Geometry: final body of the model. Coordinates: model frame, mm. Face numbers are marked on the shaded views. A direction names the side the tool comes from. Give positions to 0.01 mm unless a question says otherwise; leave off trailing zeros. Loops run counter-clockwise (first coordinate to the right, second up) from the corner with the lowest first, then second, coordinate; pieces in that order, holes last.
```python
from build123d import *
from build123d.topology import SkipClean

# Parameters (mm, degrees)
REVOLVE1_ANGLE          = 180
SKETCH12_R              = 175
BOSS_EXTRUDE2_DEPTH     = 120
BOSS_EXTRUDE2_TAPER     = 2.5
BOSS_EXTRUDE3_DEPTH     = 350
SKETCH14_R              = 112
CUT_EXTRUDE1_DEPTH      = 32
CUT_EXTRUDE1_DRAFT      = -45
SKETCH17_R              = 31
CUT_EXTRUDE3_DEPTH      = 8
SHELL1_T                = -5
SKETCH15_R              = 26
CUT_EXTRUDE2_DEPTH      = 514.054577993
BOSS_EXTRUDE4_DEPTH     = 5
BOSS_EXTRUDE5_DEPTH     = 5
ENL_V_MAT_EXTRU_2_REACH = 923.154


with BuildPart() as part:
    # Esquisse2 → Revolve1 (revolve)
    with BuildSketch(Plane.XY):
        Polygon((0, 350), (0, 0), (-47, 0), (-47, 268.593612044), align=None)
    revolve(axis=Axis((-47, 0, 0), (1, 0, 0)), revolution_arc=REVOLVE1_ANGLE)

    # Sketch12 → Boss-Extrude2 (add)
    with BuildSketch(Plane.ZY.offset(47)):
        Circle(SKETCH12_R)
    extrude(amount=BOSS_EXTRUDE2_DEPTH, taper=BOSS_EXTRUDE2_TAPER)

    # Sketch13 → Boss-Extrude3 (add)
    with BuildSketch(Plane(origin=(0, 0, 0), x_dir=(-1, 0, 0), z_dir=(0, 0, -1))):
        Polygon((0, 350), (47, 268.593612044), (47, -268.593612044), (0, -350), align=None)
    extrude(amount=BOSS_EXTRUDE3_DEPTH)


with BuildPart() as cut_extrude1_tool:
    # Sketch14 → Cut-Extrude1 (with draft: the straight prism first)
    with BuildSketch(Plane.ZY.offset(167)):
        Circle(SKETCH14_R)
    extrude(amount=-CUT_EXTRUDE1_DEPTH)
    # Cut-Extrude1: the draft: its side faces are tilted about the plane it starts from
    cut_extrude1_sides = [cut_extrude1_tool.faces().sort_by_distance(p)[0] for p in [
        (-151, 0, -112),
    ]]
    draft(cut_extrude1_sides, Plane.ZY.offset(167), CUT_EXTRUDE1_DRAFT)


with BuildPart() as part_1:
    add(part.part)

    # Cut-Extrude1: cut by cut_extrude1_tool
    add(cut_extrude1_tool.part, mode=Mode.SUBTRACT)

    # Sketch17 → Cut-Extrude3 (cut)
    with BuildSketch(Plane.ZY.offset(135)):
        Circle(SKETCH17_R)
    extrude(amount=-CUT_EXTRUDE3_DEPTH, mode=Mode.SUBTRACT)

    # Shell1
    shell1_openings = [part_1.faces().sort_by_distance(p)[0] for p in [
        (-22.469140062, 0, -350),
        (0, 0, -32.672450622),
    ]]
    offset(amount=SHELL1_T, openings=shell1_openings, kind=Kind.INTERSECTION)

    # Sketch15 → Cut-Extrude2 (cut, through all)
    with BuildSketch(Plane.ZY.offset(135)):
        Circle(SKETCH15_R)
    extrude(amount=-CUT_EXTRUDE2_DEPTH, mode=Mode.SUBTRACT)

    # Sketch18 → Revolve2 (revolve)
    with SkipClean():  # the faces are left unmerged after this step: merging them gives an invalid solid
        with BuildSketch(Plane.XY, mode=Mode.PRIVATE) as revolve2_sk:
            Polygon((-130, 82.071067812), (-89.928932188, 42), (-65, 42), (-65, 36), (-35, 36), (-35, 32), (-39, 32), (-39, 26), (-122, 26), (-122, 36), (-130, 36), align=None)
        revolve(revolve2_sk.sketch.rotate(Axis((0, 0, 0), (-1, 0, 0)), 90), axis=Axis((0, 0, 0), (-1, 0, 0)))

    # Sketch20 → Boss-Extrude4 (add)
    with SkipClean():  # the faces are left unmerged after this step: merging them gives an invalid solid
        with BuildSketch(Plane.ZY.offset(47)):
            with BuildLine():
                Line((-350, -600), (350, -600))
                Line((350, -600), (175, 0))
                ThreePointArc((175, 0), (0, -175), (-175, 0))
                Line((-175, 0), (-350, -600))
            make_face()
        extrude(amount=BOSS_EXTRUDE4_DEPTH)

    # Sketch21 → Boss-Extrude5 (add)
    with SkipClean():  # the faces are left unmerged after this step: merging them gives an invalid solid
        with BuildSketch(Plane.XZ.offset(600)):
            Polygon((-47, 350), (-47, -350), (303, -350), (478, -175), (478, 175), (303, 350), align=None)
        extrude(amount=-BOSS_EXTRUDE5_DEPTH)

    # Esquisse3 → Enlèv. mat.-Extru.2 (cut, up to next)
    with BuildSketch(Plane.ZY.offset(127), mode=Mode.PRIVATE) as enl_v_mat_extru_2_sk1:
        Polygon((-4, 30), (4, 30), (4, 26), (4, 25), (-4, 25), (-4, 26), align=None)
    enl_v_mat_extru_2_tool1 = extrude(enl_v_mat_extru_2_sk1.sketch, amount=-ENL_V_MAT_EXTRU_2_REACH, mode=Mode.PRIVATE) & part_1.part
    add(enl_v_mat_extru_2_tool1.solids().sort_by_distance((-127, 27.5, 0))[0], mode=Mode.SUBTRACT)


solid = part_1.part
```
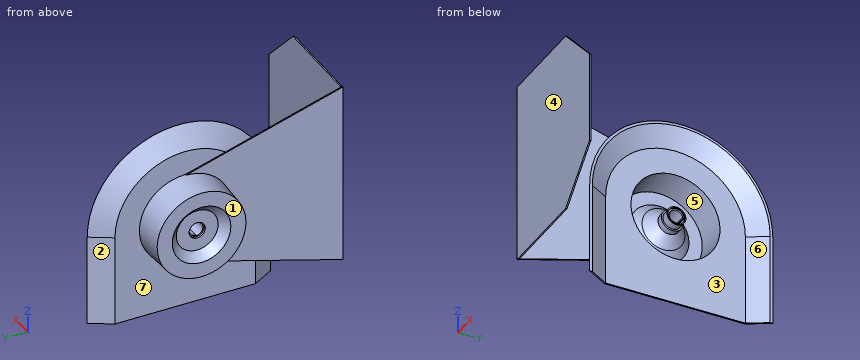
Q1. Section query A-A, the plane x = 337.5. Return loops of the section in (y, z).
Q2. Mould query, pull axis Y, two halves, no side actions, for the marked faces 1, 2, 3 and 4. Classes: +Y half, -Y half, draft (parallel to the pull), parting line (faces both ways), or undercut.
Q3. Section query B-B, the plane x = 25.5. Return loops of the section in (y, z), and give its area (3 significant figures).
Q4. Material intervals for probe 1 along Y at (x, z) = (346, 218.5); probe 2 along Y at (x, z) = (-132, 0); probe 3 along Z at (x, y) = (-94.5, -26.5), sorted ascending.
Q5. Pin query (flat end, axial travel): pin 1 Ø4.5 at (x, y) = (-98, 29) entering from +Z; pin 2 Ø10 at (x, z) = (-7.5, -111) entering from +Y; pin 3 Ø1 at (x, z) = (320, -279) entering from +Y. Return the tip coordinate at first contact, or that it passes through.
Q6. Reachability of the marked faces 5, 6 and 7 from +Z, -Z, +X, -X, +Y, -Y: full face, straight path, thin tool, end or side. Return the list, or none.
Resolved:
1. outline: (-600, -315.5) - (-595, -315.5) - (-595, 315.5) - (-600, 315.5) - close
2. face 1: draft
2. face 2: +Y half
2. face 3: undercut
2. face 4: -Y half
3. outline: (-600, -350) - (-595, -350) - (-595, 350) - (-600, 350) - close
3. area: 3,500 mm2
4. probe 1: y = -600 to -595
4. probe 2: y = -171.29 to -166.28, -84.07 to -31, 31 to 84.07, 166.28 to 171.29
4. probe 3: z = -170.88 to -165.82, -38.3 to 38.3, 165.82 to 170.88
5. pin 1: stops at z = 170.7
5. pin 2: stops at y = 345.67
5. pin 3: stops at y = -595
6. face 5: +X
6. face 6: -Z, +X
6. face 7: -X, +Y
